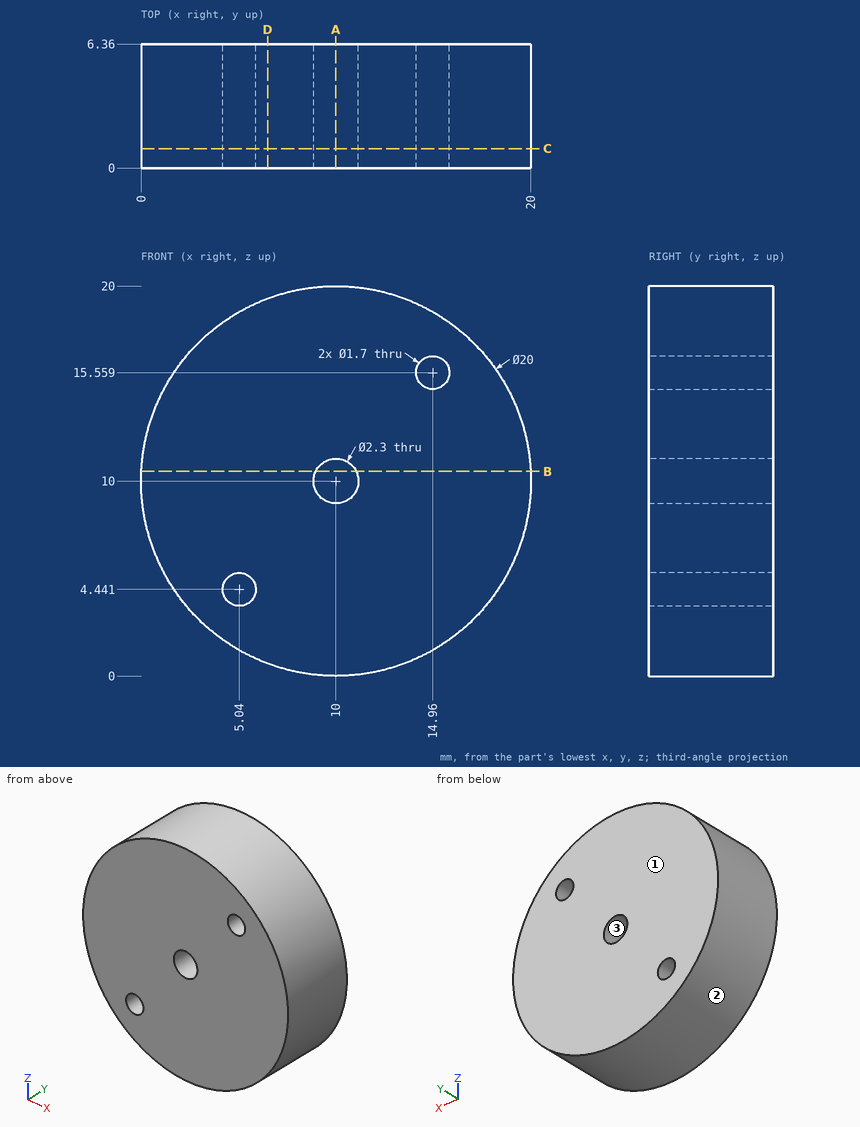
Print and shaded views of the part. All mm, measured from the part's lowest x, y and z. Coordinates: 2 decimals unless noted, no trailing zeros. Loops run counter-clockwise (first coordinate to the right, second up) from the corner with the lowest first, then second, coordinate; pieces in that order, holes last. Notation, with made-up numbers: (-1, -11) -> (21, -11) arc R26 cw to (21, 22) -> close; hole circle Ø11 at (86, 45). An arc over 180 degrees is marked (long way). Use a Markdown table: item, result. Add a question column.
Item 1: Band-saw the part on D-D on x = 6.5. Write the cut outline in (y, z).
Item 2: Band-saw the part on B-B on z = 10.5. Write the cut outline in (x, y).
Item 3: Band-saw the part on C-C on y = 1. Write the cut outline in (x, z).
Item 4: Band-saw the part on A-A on x = 10. Write the cut outline in (y, z).
Item 5: Flat gauge pins, fed straight in: P1, Ø1.4, axis at x = 14.96, z = 15.56, coming from the -Y side; P2, Ø2, axis at x = 15.5, y = 1, coming from the -Z side; P3, Ø3, axis at y = 5, z = 12, coming from the -X side; P4, Ø2, axis at x = 15.5, y = 2.5, coming from the +Z side. Where does each tip first touch, or does it go through?
Item 6: Pull direction Z, two halves, no side cores. Call the marked faces 1, 2 and 3: +Z half, -Z half, draft (parallel to the pull), parting line (faces both ways), or undercut.
Item 7: Probe probe 1 along X at (y, z) = (1.75, 10); probe 2 along Z at (x, y) = (4.75, 1.25); probe 3 along X at (y, z) = (5.75, 15.75). List the from-to ranges inside material, lowest first.
Geometry says:
| question | item | result |
|---|---|---|
| 1 | outline | (0, 0.63) -> (6.36, 0.63) -> (6.36, 19.37) -> (0, 19.37) -> close |
| 2 | outline | (0.01, 0) -> (8.96, 0) -> (8.96, 6.36) -> (0.01, 6.36) -> close; (11.04, 0) -> (19.99, 0) -> (19.99, 6.36) -> (11.04, 6.36) -> close |
| 3 | outline | circle Ø20 at (10, 10); hole circle Ø1.7 at (5.04, 4.44); hole circle Ø2.3 at (10, 10); hole circle Ø1.7 at (14.96, 15.56) |
| 4 | outline | (0, 0) -> (6.36, 0) -> (6.36, 8.85) -> (0, 8.85) -> close; (0, 11.15) -> (6.36, 11.15) -> (6.36, 20) -> (0, 20) -> close |
| 5 | P1 | through |
| 5 | P2 | z = 1.07 |
| 5 | P3 | x = 0.01 |
| 5 | P4 | z = 18.93 |
| 6 | face 1 | draft |
| 6 | face 2 | parting line |
| 6 | face 3 | undercut |
| 7 | probe 1 | 0 to 8.85, 11.15 to 20 |
| 7 | probe 2 | 1.49 to 3.64, 5.24 to 18.51 |
| 7 | probe 3 | 1.82 to 14.13, 15.79 to 18.18 |
